Input: part model. Units: mm. Frame: model coordinates. Give positions to 0.01 mm unless a question says otherwise; leave off trailing zeros. Answer as a JSON object with one key per item and string values. Group by question number.
Autodesk Inventor part; units mm, degrees
ref_plane "YZ Plane" through (0, 0, 0) normal (1, 0, 0) x (0, 1, 0)
ref_plane "XZ Plane" through (0, 0, 0) normal (0, 1, 0) x (-1, 0, 0)
ref_plane "XY Plane" through (0, 0, 0) normal (0, 0, 1) x (1, 0, 0)
sketch "Sketch1" plane through (0, 0, 0) normal (1, 0, 0) x (0, 1, 0)
  line L0 (9.5486, -7.0751) -> (4.5486, -7.0751)
  line L1 (7.0486, -9.5751) -> (7.0486, -4.5751)
  circle A0 centre (7.0486, -7.0751) radius 2
  circle A1 centre (7.0486, 6.9249) radius 2
  line L2 (7.0486, 9.4249) -> (7.0486, 4.4249)
  line L3 (9.5486, 6.9249) -> (4.5486, 6.9249)
  line L4 (4.1986, 4.8676) -> (4.1986, 8.1249)
  arc A2 (4.1986, 8.1249) -> (3.8986, 8.4249) centre (3.8986, 8.1249) ccw
  line L5 (3.8986, 8.4249) -> (2.9986, 8.4249)
  arc A3 (2.6986, 8.7249) -> (2.9986, 8.4249) centre (2.9986, 8.7249) ccw
  line L6 (2.6986, 8.7249) -> (2.6986, 9.6249)
  arc A4 (2.9986, 9.9249) -> (2.6986, 9.6249) centre (2.9986, 9.6249) ccw
  line L7 (2.9986, 9.9249) -> (9.7486, 9.9249)
  arc A5 (10.0486, 9.6249) -> (9.7486, 9.9249) centre (9.7486, 9.6249) ccw
  line L8 (10.0486, 9.6249) -> (10.0486, 2.8749)
  arc A6 (9.7486, 2.5749) -> (10.0486, 2.8749) centre (9.7486, 2.8749) ccw
  line L9 (9.7486, 2.5749) -> (8.8486, 2.5749)
  arc A7 (8.5486, 2.8749) -> (8.8486, 2.5749) centre (8.8486, 2.8749) ccw
  line L10 (8.5486, 2.8749) -> (8.5486, 3.7749)
  arc A8 (8.5486, 3.7749) -> (8.2486, 4.0749) centre (8.2486, 3.7749) ccw
  line L11 (8.2486, 4.0749) -> (4.9914, 4.0749)
  arc A9 (4.9914, 4.0749) -> (4.7564, 3.9614) centre (4.9914, 3.7749) ccw
  arc A10 (4.7564, 3.9614) -> (3.3559, 0.2322) centre (9.8395, -0.0751) ccw
  line L12 (3.3559, 0.2322) -> (3.0486, -0.0751)
  line L13 (3.0486, -0.0751) -> (3.3559, -0.3824)
  arc A11 (3.3559, -0.3824) -> (4.7564, -4.1117) centre (9.8395, -0.0751) ccw
  arc A12 (4.7564, -4.1117) -> (4.9914, -4.2251) centre (4.9914, -3.9251) ccw
  line L14 (4.9914, -4.2251) -> (8.2486, -4.2251)
  arc A13 (8.2486, -4.2251) -> (8.5486, -3.9251) centre (8.2486, -3.9251) ccw
  line L15 (8.5486, -3.9251) -> (8.5486, -3.0251)
  arc A14 (8.8486, -2.7251) -> (8.5486, -3.0251) centre (8.8486, -3.0251) ccw
  line L16 (8.8486, -2.7251) -> (9.7486, -2.7251)
  arc A15 (10.0486, -3.0251) -> (9.7486, -2.7251) centre (9.7486, -3.0251) ccw
  line L17 (10.0486, -3.0251) -> (10.0486, -9.7751)
  arc A16 (9.7486, -10.0751) -> (10.0486, -9.7751) centre (9.7486, -9.7751) ccw
  line L18 (9.7486, -10.0751) -> (2.9986, -10.0751)
  arc A17 (2.6986, -9.7751) -> (2.9986, -10.0751) centre (2.9986, -9.7751) ccw
  line L19 (2.6986, -9.7751) -> (2.6986, -8.8751)
  arc A18 (2.9986, -8.5751) -> (2.6986, -8.8751) centre (2.9986, -8.8751) ccw
  line L20 (2.9986, -8.5751) -> (3.8986, -8.5751)
  arc A19 (3.8986, -8.5751) -> (4.1986, -8.2751) centre (3.8986, -8.2751) ccw
  line L21 (4.1986, -8.2751) -> (4.1986, -5.0179)
  arc A20 (4.1986, -5.0179) -> (4.0852, -4.7829) centre (3.8986, -5.0179) ccw
  arc A21 (4.0852, -4.7829) -> (0.3559, -3.3824) centre (0.0486, -9.8659) ccw
  line L22 (0.3559, -3.3824) -> (0.0486, -3.0751)
  line L23 (0.0486, -3.0751) -> (-0.2587, -3.3824)
  arc A22 (-0.2587, -3.3824) -> (-3.9879, -4.7829) centre (0.0486, -9.8659) ccw
  arc A23 (-3.9879, -4.7829) -> (-4.1014, -5.0179) centre (-3.8014, -5.0179) ccw
  line L24 (-4.1014, -5.0179) -> (-4.1014, -8.2751)
  arc A24 (-4.1014, -8.2751) -> (-3.8014, -8.5751) centre (-3.8014, -8.2751) ccw
  line L25 (-3.8014, -8.5751) -> (-2.9014, -8.5751)
  arc A25 (-2.6014, -8.8751) -> (-2.9014, -8.5751) centre (-2.9014, -8.8751) ccw
  line L26 (-2.6014, -8.8751) -> (-2.6014, -9.7751)
  arc A26 (-2.9014, -10.0751) -> (-2.6014, -9.7751) centre (-2.9014, -9.7751) ccw
  line L27 (-2.9014, -10.0751) -> (-9.6514, -10.0751)
  arc A27 (-9.9514, -9.7751) -> (-9.6514, -10.0751) centre (-9.6514, -9.7751) ccw
  line L28 (-9.9514, -9.7751) -> (-9.9514, -3.0251)
  arc A28 (-9.6514, -2.7251) -> (-9.9514, -3.0251) centre (-9.6514, -3.0251) ccw
  line L29 (-9.6514, -2.7251) -> (-8.7514, -2.7251)
  arc A29 (-8.4514, -3.0251) -> (-8.7514, -2.7251) centre (-8.7514, -3.0251) ccw
  line L30 (-8.4514, -3.0251) -> (-8.4514, -3.9251)
  arc A30 (-8.4514, -3.9251) -> (-8.1514, -4.2251) centre (-8.1514, -3.9251) ccw
  line L31 (-8.1514, -4.2251) -> (-4.8941, -4.2251)
  arc A31 (-4.8941, -4.2251) -> (-4.6592, -4.1117) centre (-4.8941, -3.9251) ccw
  arc A32 (-4.6592, -4.1117) -> (-3.2587, -0.3824) centre (-9.7422, -0.0751) ccw
  line L32 (-3.2587, -0.3824) -> (-2.9514, -0.0751)
  line L33 (-2.9514, -0.0751) -> (-3.2587, 0.2322)
  arc A33 (-3.2587, 0.2322) -> (-4.6592, 3.9614) centre (-9.7422, -0.0751) ccw
  arc A34 (-4.6592, 3.9614) -> (-4.8941, 4.0749) centre (-4.8941, 3.7749) ccw
  line L34 (-4.8941, 4.0749) -> (-8.1514, 4.0749)
  arc A35 (-8.1514, 4.0749) -> (-8.4514, 3.7749) centre (-8.1514, 3.7749) ccw
  line L35 (-8.4514, 3.7749) -> (-8.4514, 2.8749)
  arc A36 (-8.7514, 2.5749) -> (-8.4514, 2.8749) centre (-8.7514, 2.8749) ccw
  line L36 (-8.7514, 2.5749) -> (-9.6514, 2.5749)
  arc A37 (-9.9514, 2.8749) -> (-9.6514, 2.5749) centre (-9.6514, 2.8749) ccw
  line L37 (-9.9514, 2.8749) -> (-9.9514, 9.6249)
  arc A38 (-9.6514, 9.9249) -> (-9.9514, 9.6249) centre (-9.6514, 9.6249) ccw
  line L38 (-9.6514, 9.9249) -> (-2.9014, 9.9249)
  arc A39 (-2.6014, 9.6249) -> (-2.9014, 9.9249) centre (-2.9014, 9.6249) ccw
  line L39 (-2.6014, 9.6249) -> (-2.6014, 8.7249)
  arc A40 (-2.9014, 8.4249) -> (-2.6014, 8.7249) centre (-2.9014, 8.7249) ccw
  line L40 (-2.9014, 8.4249) -> (-3.8014, 8.4249)
  arc A41 (-3.8014, 8.4249) -> (-4.1014, 8.1249) centre (-3.8014, 8.1249) ccw
  line L41 (-4.1014, 8.1249) -> (-4.1014, 4.8676)
  arc A42 (-4.1014, 4.8676) -> (-3.9879, 4.6327) centre (-3.8014, 4.8676) ccw
  arc A43 (-3.9879, 4.6327) -> (-0.2587, 3.2322) centre (0.0486, 9.7157) ccw
  line L42 (-0.2587, 3.2322) -> (0.0486, 2.9249)
  line L43 (0.0486, 2.9249) -> (0.3559, 3.2322)
  arc A44 (0.3559, 3.2322) -> (4.0852, 4.6327) centre (0.0486, 9.7157) ccw
  arc A45 (4.0852, 4.6327) -> (4.1986, 4.8676) centre (3.8986, 4.8676) ccw
  line L44 (-11.1503, -0.0751) -> (11.2475, -0.0751)
  circle A46 centre (0.0486, -0.0751) radius 2.15
  circle A47 centre (-6.9514, -7.0751) radius 2
  line L45 (-6.9514, -9.5751) -> (-6.9514, -4.5751)
  line L46 (-9.4514, -7.0751) -> (-4.4514, -7.0751)
  circle A48 centre (-6.9514, 6.9249) radius 2
  line L47 (-6.9514, 9.4249) -> (-6.9514, 4.4249)
  line L48 (-9.4514, 6.9249) -> (-4.4514, 6.9249)
extrude "Extrusion1" add sketch "Sketch1" along normal blind 470
equation "\"BendRadius\" = Thickness"
equation "\"BendReliefWidth\" = Thickness"
equation "\"BendReliefDepth\" = 0.5 * Thickness"
equation "\"CornerReliefSize\" = 4 * Thickness"
equation "\"MinimumRemnant\" = 2 * Thickness"
equation "\"TransitionRadius\" = BendRadius"
equation "\"JacobiRadiusSize\" = BendRadius"
equation "\"GapSize\" = Thickness"
properties part number "600mm 2020"
1) Cut plane A-A on x = 433. Count the separate pieces of the cut face and the enclosed holes in it, and give its area (3 significant figures).
2) Line query: line 1 along Y through (x, z) = (302, 6.5); line 2 along Z through (x, y) = (40.5, 3); line 3 along Y through (x, z) = (175, 2.75). Output: solid intervals per line, ascending. Write a range as from..to.
3) Pin query (flat end, axial travel): P1, Ø1.5, axis at y = 7.5, z = 0.5, coming from the -X side. Return the tip coordinate at first contact, or that it passes through.
Filled in:
{
 "1": {"separate pieces": "1", "enclosed holes": "4", "area": "160 mm²"},
 "2": {"line 1": "y = -9.95..-8.91, -5..-4.1, 4.2..5.09, 9..10.05", "line 2": "z = -10.08..-8.58, -4.08..3.93, 8.42..9.92", "line 3": "y = -9.92..-8.48, -3.9..4, 8.58..10.02"},
 "3": {"P1": "passes through"}
}
